Could you check a few things on this model? Use its own coordinates, in mm. A direction names the side the tool comes from. Round coordinates to 2 decimals unless told otherwise and drop trailing zeros. Loops run counter-clockwise (first coordinate to the right, second up) from the corner with the lowest first, then second, coordinate; pieces in that order, holes last. Notation, with made-up numbers: M 39.5,15.5 L 83.5,15.5 A17 ccw 83.5,40.5 Z; hole C -32,26.25 d7. An arc over 180 degrees is marked long. Answer in a Markdown table with one row per item.
Autodesk Inventor part; units mm, degrees
ref_plane "YZ Plane" through (0, 0, 0) normal (1, 0, 0) x (0, 1, 0)
ref_plane "XZ Plane" through (0, 0, 0) normal (0, 1, 0) x (-1, 0, 0)
ref_plane "XY Plane" through (0, 0, 0) normal (0, 0, 1) x (1, 0, 0)
sketch "Sketch1" plane through (0, 0, 0) normal (0, 0, 1) x (1, 0, 0)
  line L0 (-40, -4.6078) -> (40, -4.6078)
  line L1 (40, -4.6078) -> (40, 38.3746)
  line L2 (-40, 38.3746) -> (-40, -4.6078)
  line L3 (-40, 59.3419) -> (-40, 38.3746)
  line L4 (40, 59.3419) -> (40, 38.3746)
  line L5 (-40, 59.3419) -> (0, 74.1322)
  line L6 (0, 74.1322) -> (40, 59.3419)
  point P0 (0, 0)
  dimension "d0" = 80
  dimension "d5" = 78.74
extrude "Extrusion1" add sketch "Sketch1" along normal blind 50.8
sketch "Sketch4" plane through (0, 0, 50.8) normal (0, 0, 1) x (1, 0, 0)
  line L0 (-27.6156, 7.8338) -> (-12.3756, 7.8338)
  line L1 (-12.3756, 7.8338) -> (-12.3756, 24.8882)
  line L2 (-12.3756, 24.8882) -> (-27.6156, 24.8882)
  line L3 (-27.6156, 24.8882) -> (-27.6156, 7.8338)
  line L4 (-7.2956, 7.8338) -> (7.9444, 7.8338)
  line L5 (7.9444, 7.8338) -> (7.9444, 24.8882)
  line L6 (7.9444, 24.8882) -> (-7.2956, 24.8882)
  line L7 (-7.2956, 24.8882) -> (-7.2956, 7.8338)
  line L8 (13.0244, 7.8338) -> (28.2644, 7.8338)
  line L9 (28.2644, 7.8338) -> (28.2644, 24.8882)
  line L10 (28.2644, 24.8882) -> (13.0244, 24.8882)
  line L11 (13.0244, 24.8882) -> (13.0244, 7.8338)
  point P0 (0, 0)
  dimension "d17" = 15.24
  dimension "d19" = 15.24
  dimension "d21" = 15.24
extrude "Extrusion2" add sketch "Sketch4" along normal blind 25.4
properties part number "cwsumorobot"
1) Which directions (+Z, -Z, +X, -X, +Y, -Y) give clear straight access to the entire face, cutting with the end or side of a thin tool? Please do faces 5 (the face through (-27.616, 16, 63)), 6 (the face through (0, 7.834, 63)), 7 (the face through (7.944, 16, 63)), 8 (the face through (-20, 24.888, 63)).
Computed:
| item | result |
|---|---|
| face 5 | +Z, -X, +Y, -Y |
| face 6 | +Z, +X, -X, -Y |
| face 7 | +Z, +Y, -Y |
| face 8 | +Z, +X, -X, +Y |
2) I want a section at A-A, the plane z = 64.5. Please give me the cut outline in (x, y), plus the area to 3 significant figures.
Computed:
| item | result |
|---|---|
| outline | M -27.62,7.83 L -12.38,7.83 L -12.38,24.89 L -27.62,24.89 Z; M -7.3,7.83 L 7.94,7.83 L 7.94,24.89 L -7.3,24.89 Z; M 13.02,7.83 L 28.26,7.83 L 28.26,24.89 L 13.02,24.89 Z |
| area | 780 mm² |
3) I want a section at D-D, the plane z = 38. Please give me the cut outline in (x, y).
Computed:
| item | result |
|---|---|
| outline | M -40,-4.61 L 40,-4.61 L 40,59.34 L 0,74.13 L -40,59.34 Z |
4) I want a section at C-C, the plane x = 17. Please give me the cut outline in (y, z), plus the area to 3 significant figures.
Computed:
| item | result |
|---|---|
| outline | M -4.61,0 L 67.85,0 L 67.85,50.8 L 24.89,50.8 L 24.89,76.2 L 7.83,76.2 L 7.83,50.8 L -4.61,50.8 Z |
| area | 4,110 mm² |
5) Will these pins go through, and if not, where does the flat tip stop? P1, Ø5, axis at y = 20, z = 58, coming from the -X side; P2, Ø4.5, axis at x = -20, z = 58.5, coming from the -Y side; P3, Ø4.5, axis at x = 23.5, z = 59.5, coming from the +Y side.
Computed:
| item | result |
|---|---|
| P1 | stops at x = -27.62 |
| P2 | stops at y = 7.83 |
| P3 | stops at y = 24.89 |
6) I need wall thicknesses on line 1 (X direction, y = 11.5, z = 63.5); line 2 (Z direction, x = 30, y = 19); line 3 (Y direction, x = -26, z = 68). Which ranges of each line are inside material? Lowest first, please.
Computed:
| item | result |
|---|---|
| line 1 | x = -27.62 to -12.38, -7.3 to 7.94, 13.02 to 28.26 |
| line 2 | z = 0 to 50.8 |
| line 3 | y = 7.83 to 24.89 |
7) If we mould it in two halves opening along X, with no side actions, what happens to faces 1 (the face through (19.72, 66.84, 25.04)), 2 (the face through (-20, 16, 76.2)), 3 (the face through (13.024, 16, 63)), 4 (the face through (-12.376, 16, 63))? For each: released by +X, released by -X, zero draft, split by the parting line, or undercut.
Computed:
| item | result |
|---|---|
| face 1 | released by +X |
| face 2 | zero draft |
| face 3 | undercut |
| face 4 | undercut |
8) I want a section at B-B, the plane y = 17.5. Please give me the cut outline in (x, z), plus the area to 3 significant figures.
Computed:
| item | result |
|---|---|
| outline | M -40,0 L 40,0 L 40,50.8 L 28.26,50.8 L 28.26,76.2 L 13.02,76.2 L 13.02,50.8 L 7.94,50.8 L 7.94,76.2 L -7.3,76.2 L -7.3,50.8 L -12.38,50.8 L -12.38,76.2 L -27.62,76.2 L -27.62,50.8 L -40,50.8 Z |
| area | 5,230 mm² |
